For this review, use the dimensioned drawing (mm, ordinates from the lowest corner) and the shaded views. A direction names the side the tool comes from. Give positions to 0.01 mm unless a question says otherwise; leave off trailing zeros. Loops run counter-clockwise (first coordinate to the right, second up) from the corner with the lowest first, then second, coordinate; pieces in that order, holes last. Notation, with made-up numbers: M -32,-7 L -18,-7 A16 ccw -18,1 Z; hole C 60,83 d9. An arc over 180 degrees is marked long. Return JSON: item names as keys, results as strings.
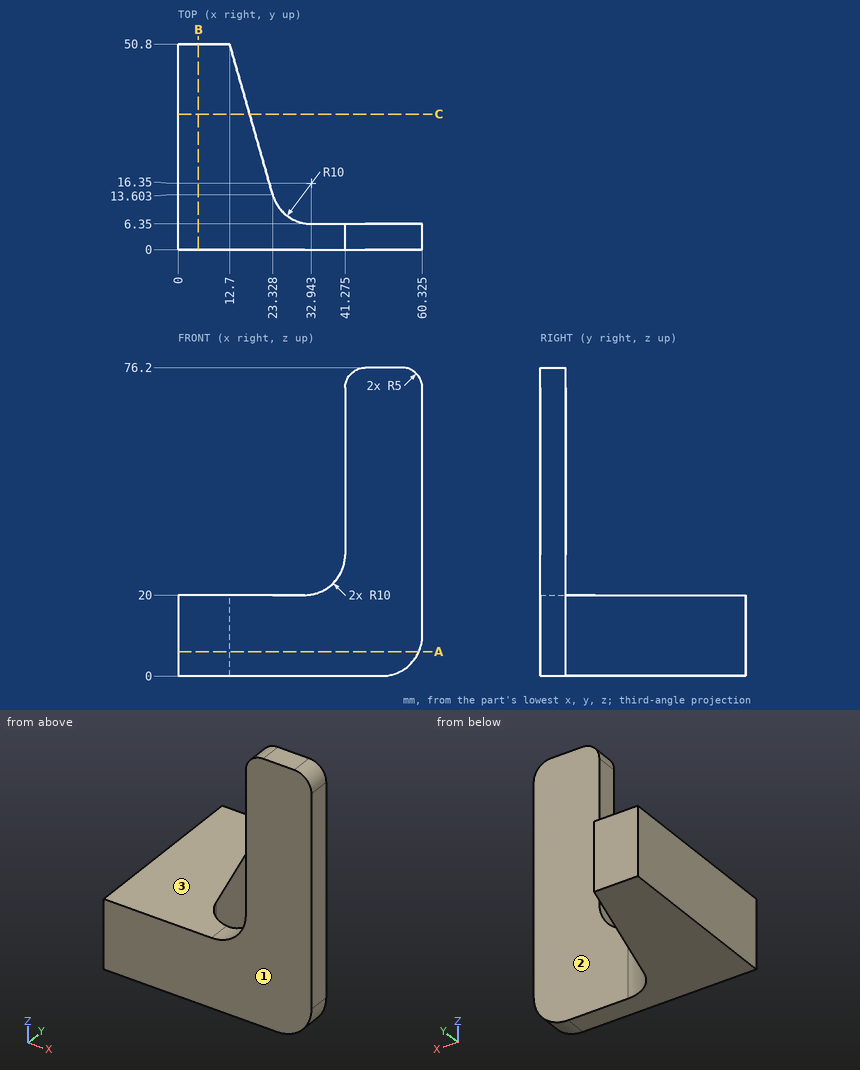
1) Consider section B-B on x = 5. Write out the cut boundary in (y, z).
From the geometry:
{"outline": "M 0,0 L 50.8,0 L 50.8,20 L 0,20 Z"}
2) Wall thickness on L1, parallel to Z at x = 10, y = 36.5; L2, parallel to X at y = 4, z = 48 (3 decimals); L3, parallel to Y at x = 55, z = 14.5: over which ranges is each line inside the solid? List them lowest first. Write a range as from..to.
From the geometry:
{"L1": "0..20", "L2": "41.275..60.325", "L3": "0..6.35"}
3) Tool access review of the marked faces 1, 2 and 3: name each direction out of +Z, -Z, +X, -X, +Y, -Y from which nothing blocks a thin tool from reaching the whole face with its end or side.
From the geometry:
{"face 1": "+Z, -Z, +X, -X, -Y", "face 2": "+Z, -Z, +X, +Y", "face 3": "+Z, -X, +Y, -Y"}
4) Consider section A-A on z = 6. Write out the cut boundary in (x, y), then the cut area to 3 significant figures.
From the geometry:
{"outline": "M 0,0 L 59.49,0 L 59.49,6.35 L 32.94,6.35 A10 cw 23.33,13.6 L 12.7,50.8 L 0,50.8 Z", "area": "1,240 mm²"}
5) Consider section C-C on y = 33.5. Write out the cut boundary in (x, z), then the cut area to 3 significant figures.
From the geometry:
{"outline": "M 0,0 L 17.64,0 L 17.64,20 L 0,20 Z", "area": "353 mm²"}
6) Insertion check: pin 1 (3 mm diameter, centred on y = 3.5, z = 55.5, fed in from -X) (3 decimals); pin 2 (22 mm diameter, centred on x = 45.5, z = 25.5, fed in from +Y). Each pin has a flat end and moves straight along its axis. Give the tip position at first contact, or say it passes through.
From the geometry:
{"pin 1": "x = 41.275", "pin 2": "y = 6.35"}
